from build123d import *

# Parameters (mm, degrees)
BOSS_EXTRUDE1_DEPTH      = 20
BOSS_EXTRUDE2_DEPTH      = 5
BOSS_EXTRUDE2_DEPTH_BACK = 5
SKETCH3_R                = 10
SKETCH3_R_2              = 5
BOSS_EXTRUDE3_DEPTH      = 2.5
BOSS_EXTRUDE3_DEPTH_BACK = 2.5
SKETCH4_W                = 9.507770028
SKETCH4_H                = 1.347875139
MOVE_FACE1_BY            = 11.3
BODY_MOVE_COPY2_ANGLE    = 60
BODY_MOVE_COPY3_ANGLE    = 180


with BuildPart() as part:
    # Sketch1 → Boss-Extrude1 (new body)
    with BuildSketch(Plane(origin=(0, 0, 0), x_dir=(1, 0, 0), z_dir=(0, 1, 0))):
        Polygon((-36.5, 6.780145524), (36.5, 6.780145524), (0, 70), align=None)
    extrude(amount=BOSS_EXTRUDE1_DEPTH)


with BuildPart() as body_2:
    # Sketch3 → Boss-Extrude2 (new, two sides: drawn at the far end of the back side and taken through both)
    with BuildSketch(Plane(origin=(0, 0, 0), x_dir=(0, -1, 0), z_dir=(-1, 0, 0)).offset(-BOSS_EXTRUDE2_DEPTH_BACK)):
        with Locations(Location((-10.287349531, -80, 0), (0, 0, 90))):
            Circle(SKETCH3_R)
        with Locations(Location((-10.287349531, -80, 0), (0, 0, 90))):
            Circle(SKETCH3_R_2, mode=Mode.SUBTRACT)
    extrude(amount=BOSS_EXTRUDE2_DEPTH + BOSS_EXTRUDE2_DEPTH_BACK)

    # Sketch4 → Boss-Extrude3 (add, two sides: drawn at the far end of the back side and taken through both)
    with BuildSketch(Plane(origin=(0, 0, 0), x_dir=(0, -1, 0), z_dir=(-1, 0, 0)).offset(-BOSS_EXTRUDE3_DEPTH_BACK)):
        with Locations((-10, -70.673937569)):
            Rectangle(SKETCH4_W, SKETCH4_H)
    extrude(amount=BOSS_EXTRUDE3_DEPTH + BOSS_EXTRUDE3_DEPTH_BACK)

    # Move Face1: a face moved outward by 11.3
    extrude(body_2.faces().sort_by_distance((0, 10, -70))[0], amount=MOVE_FACE1_BY, dir=(0, 0, 1))


with BuildPart() as body_3:
    # Body-Move/Copy1: copy of body 2
    add(body_2.part.moved(Location((50, 0, 0))))


with BuildPart() as body_3_1:
    # Body-Move/Copy2: read off the stored shape, not the designer's step
    # Body-Move/Copy2: moved
    add(body_3.part.moved(Location((-25.8782217, 0, 45.4663337))).rotate(Axis((0, 0, 0), (0, 1, 0)), BODY_MOVE_COPY2_ANGLE))


with BuildPart() as body_3_2:
    # Body-Move/Copy3: moved
    add(body_3_1.part.rotate(Axis((-13.578099639, 0, -36.414437667), (0, 1, 0)), BODY_MOVE_COPY3_ANGLE))


with BuildPart() as body_3_3:
    # Body-Move/Copy4: moved
    add(body_3_2.part.moved(Location((60.621778265, 0, 35))))


with BuildPart() as body_3_4:
    # Body-Move/Copy5: read off the stored shape, not the designer's step
    # Body-Move/Copy5: moved
    add(body_3_3.part.moved(Location((-5.5290056, 0, -3.1921729))))


with BuildPart() as body_3_5:
    # Body-Move/Copy6: read off the stored shape, not the designer's step
    # Body-Move/Copy6: moved
    add(body_3_4.part.moved(Location((-0.625, 0, 1.0825318))))


with BuildPart() as body_4:
    # Mirror1: mirrored copy
    add(body_3_5.part.mirror(Plane.ZY))


with BuildPart() as part_1:
    add(part.part)

    # Combine1: union body 2, body 3, body 4
    add(body_2.part)
    add(body_3_5.part)
    add(body_4.part)


solid = part_1.part
Can you work these out from the model? Positions are in its coordinate system, mm. A direction names the side the tool comes from. Give positions to 0.01 mm unless a question says otherwise; leave off trailing zeros. Order: outer loops, then holes, each group sorted by start corner. A loop starts at its lowest first (then second) coordinate and runs counter-clockwise, first axis right, second up. Notation, with made-up numbers: M 40,48.25 L 91,48.25 A27 cw 91,82.25 Z; hole C -28.75,11.5 d9. An arc over 180 degrees is marked long. Use one line per item in the form item = value. Start each with the question number.
Item 1: Will these pins go through, and if not, where does the flat tip stop? pin 1 Ø1.7 at (y, z) = (9, -67.5) entering from +X; pin 2 Ø8 at (y, z) = (9.5, -33.5) entering from -X; pin 3 Ø1.5 at (x, y) = (32, 8.5) entering from +Z.
Item 2: If we section it at A-A (z = -80): Write out the boundary of the cut face in (x, y).
Item 3: If I drill on line 1 along Y through (x, z) = (2, -80); line 2 along X through (y, z) = (14.5, 0); line 3 along Y through (x, z) = (-8.5, -49), over which ranges is the centre line in solid material (lowest first)?
Item 4: If we section it at D-D (z = -49): Write out the boundary of the cut face in (x, y), then the cut area to 3 significant figures.
Item 5: We'd pull the mould along Y, two halves only. Please class faces 1 (the flat face through (1, 5.246, -69)), 2 (the flat face through (18.505, 9.86, -37.948)), 3 (the cylindrical face through (41.123, 8.372, -4.03)): +Y half, -Y half, draft (parallel to the pull), parting line (faces both ways), or undercut.
Item 6: If we section it at B-B (y = 18.5): Write out the boundary of the cut face in (x, z).
Item 7: If we section it at C-C (x = -9.5): Write out the boundary of the cut face in (y, z), then the cut area to 3 significant figures.
Item 8: For faces 4 (the flat face through (5, 8, -85)), 5 (the flat face through (-1, 20, -32)), 6 (the flat face through (44.703, 14.872, 3.73)), which set-ups out of +Z, -Z, +X, -X, +Y, -Y let a thin tool reach every point of the face, with its end or its side?
Outcome:
q1.pin_1 = 2.5
q1.pin_2 = -23.38
q1.pin_3 = -6.06
q2.outline = M -5,0.29 L 5,0.29 L 5,5.29 L -5,5.29 Z; M -5,15.29 L 5,15.29 L 5,20.29 L -5,20.29 Z
q3.line_1 = 0.29 to 5.29, 15.29 to 20.29
q3.line_2 = -54.6 to -47.24, -41.02 to -38.24, 38.24 to 41.02, 47.24 to 54.6
q3.line_3 = 0 to 20
q4.outline = M -12.12,0 L 12.12,0 L 12.12,20 L -12.12,20 Z
q4.area = 485 mm2
q5.face_1 = -Y half
q5.face_2 = draft
q5.face_3 = undercut
q6.outline = M -52.6,-3.26 L -42.72,-8.96 L -37.72,-0.3 L -47.6,5.4 Z; M -36.5,-6.78 L 0,-70 L 36.5,-6.78 Z; M -5,-85.71 L 5,-85.71 L 5,-74.29 L -5,-74.29 Z; M 37.72,-0.3 L 42.72,-8.96 L 52.6,-3.26 L 47.6,5.4 Z
q7.outline = M 0,-53.55 L 20,-53.55 L 20,-6.78 L 0,-6.78 Z
q7.area = 935 mm2
q8.face_4 = -Z, +X, +Y, -Y
q8.face_5 = +Z, +X, -X, +Y
q8.face_6 = +Z, +Y, -Y
